Design review of the part built by this model. Coordinates are the model's own, in mm. Give positions to 0.01 mm unless a question says otherwise; leave off trailing zeros. Write each loop counter-clockwise with the first axis right and the second up, starting at its lowest first coordinate (ties: lowest second). Pieces come first, ordered by that corner, then holes. Notation, with made-up numbers: (50, 70.5) -> (79, 70.5) arc R18 cw to (79, 80.5) -> close; hole circle Ø10 at (68, 74.5). An arc over 180 degrees is marked (long way). Write each question's results on one line, items separated by ' | '. Start each with the question number.
(1) Take a section at A-A (y = 1.4). State the section outline as (x, z) points.
(2) To check wall thickness, follow probe 1 along Z at (x, y) = (-14.5, 1.65); probe 2 along Z at (x, y) = (-9, 0.3); probe 3 along X at (y, z) = (1.45, -15). State the ranges of each line that lie inside material, in increasing order.
(3) Clearance check with a flat-ended pin moving along its axis: pin 1 (4 mm diameter, centred on x = 13, z = -12, fed in from +Y). State where the tip first meets the part, or that it passes through.
from build123d import *

# Parameters (mm, degrees)
SKETCH1_R           = 17.25
BOSS_EXTRUDE1_DEPTH = 2
SKETCH2_OUTSIDE_W   = 46.266
SKETCH2_OUTSIDE_H   = 46.266
SKETCH2_OUTSIDE_R   = 17
CUT_EXTRUDE1_DEPTH  = 1
CHAMFER1_SIZE       = 0.2


with BuildPart() as part:
    # Sketch1 → Boss-Extrude1 (new body)
    with BuildSketch(Plane(origin=(0, 0, 0), x_dir=(1, 0, 0), z_dir=(0, 1, 0))):
        with Locations(Location((0, 0, 0), (0, 0, 270))):
            Circle(SKETCH1_R)
    extrude(amount=BOSS_EXTRUDE1_DEPTH)

    # Sketch2 outside → Cut-Extrude1 (cut)
    with BuildSketch(Plane(origin=(0, 2, 0), x_dir=(1, 0, 0), z_dir=(0, 1, 0))):
        Rectangle(SKETCH2_OUTSIDE_W, SKETCH2_OUTSIDE_H)
        with Locations(Location((0, 0, 0), (0, 0, 270))):
            Circle(SKETCH2_OUTSIDE_R, mode=Mode.SUBTRACT)
    extrude(amount=-CUT_EXTRUDE1_DEPTH, mode=Mode.SUBTRACT)

    # Chamfer1
    chamfer1_edges = [part.edges().sort_by_distance(p)[0] for p in [
        (0, 2, -17),
        (0, 0, -17.25),
    ]]
    chamfer(chamfer1_edges, length=CHAMFER1_SIZE)


solid = part.part
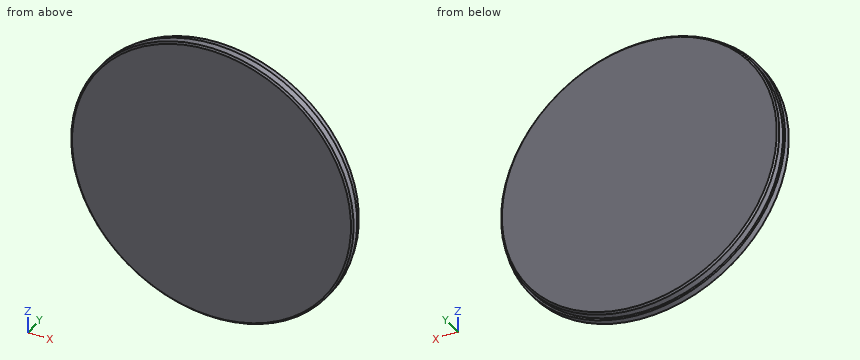
Report:
1) outline: circle Ø34 at (0, 0)
2) probe 1: -8.87 to 8.87 | probe 2: -14.72 to 14.72 | probe 3: -8 to 8
3) pin 1: y = 2
